```python
from build123d import *

# Parameters (mm, degrees)
F1_DEPTH = 25
F2_W     = 5
F2_H     = 25
F3_DEPTH = 5
F4_SIZE  = 2
F5_R     = 2
F6_R     = 5


with BuildPart() as f1:
    # F0 (on Top) → F1 (new body)
    with BuildSketch(Plane.XY):
        with BuildLine():
            ThreePointArc((57.667806, -47.952312), (0, -75), (-57.667806, -47.952312))
            Line((-57.667806, -47.952312), (-88.564008, -82.249977))
            Line((-88.564008, -82.249977), (0, -82.249977))
            Line((0, -82.249977), (88.564008, -82.249977))
            Line((88.564008, -82.249977), (57.667806, -47.952312))
        make_face()
    extrude(amount=F1_DEPTH)

    # F2 (on face) → F3 (join)
    with BuildSketch(Plane.XZ.offset(82.249977)):
        with Locations((77.608379, 12.5)):
            Rectangle(F2_W, F2_H)
        with Locations((-77.608379, 12.5)):
            Rectangle(F2_W, F2_H)
    extrude(amount=F3_DEPTH)

    # F4
    f4_edges = [f1.edges().sort_by_distance(p)[0] for p in [
        (-80.108379, -87.249977, 12.5),
        (-75.108379, -87.249977, 12.5),
        (75.108379, -87.249977, 12.5),
        (80.108379, -87.249977, 12.5),
    ]]
    chamfer(f4_edges, length=F4_SIZE)

    # F5
    f5_edges = [f1.edges().sort_by_distance(p)[0] for p in [
        (-80.108379, -82.249977, 12.5),
        (-75.108379, -82.249977, 12.5),
        (80.108379, -82.249977, 12.5),
        (75.108379, -82.249977, 12.5),
        (57.667806, -47.952312, 12.5),
        (-57.667806, -47.952312, 12.5),
    ]]
    fillet(f5_edges, radius=F5_R)

    # F6
    f6_edges = [f1.edges().sort_by_distance(p)[0] for p in [
        (-88.564008, -82.249977, 12.5),
        (88.564008, -82.249977, 12.5),
    ]]
    fillet(f6_edges, radius=F6_R)


solid = f1.part
```
Verification items for the finished model (mm, model axes). A direction names the side the tool comes from. Round coordinates to 2 decimals unless told otherwise and drop trailing zeros. Write each loop counter-clockwise with the first axis right and the second up, starting at its lowest first coordinate (ties: lowest second). Pieces come first, ordered by that corner, then holes. Notation, with made-up numbers: (-36.5, -25) -> (8.5, -25) arc R19 cw to (8.5, -4) -> close; hole circle Ø6 at (49.25, 69). An arc over 180 degrees is marked (long way). Write each question's results on one line, items separated by ' | '.
Q1. Sectioned sample at D-D, the plane x = 16.5. Record the boundary of the cut face in (y, z).
Derived:
outline: (-82.25, 0) -> (-73.16, 0) -> (-73.16, 25) -> (-82.25, 25) -> close
Q2. Sectioned sample at B-B, the plane y = -66. Record the boundary of the cut face in (x, z), and give its area (3 significant figures).
Derived:
outline: (-73.93, 0) -> (-35.62, 0) -> (-35.62, 25) -> (-73.93, 25) -> close; (35.62, 0) -> (73.93, 0) -> (73.93, 25) -> (35.62, 25) -> close | area: 1,920 mm²
Q3. Thickness scan on probe 1 along X at (y, z) = (-85, 18.5); probe 2 along X at (y, z) = (-59, 11.75); probe 3 along Y at (x, z) = (-58, 12). Record the ranges inside material, lowest first.
Derived:
probe 1: x = -80.11 to -75.11, 75.11 to 80.11 | probe 2: x = -67.62 to -46.3, 46.3 to 67.62 | probe 3: y = -82.25 to -49
Q4. Draft check along X on faces 1 (the face through (-1, -76, 0)), 2 (the face through (57.672, -48.982, 12.675)), 3 (the face through (70.777, -62.505, 12.325)), 4 (the face through (-70.46, -62.15, 12.32)). Enter one of: released by +X, released by -X, zero draft, split by the parting line, or undercut.
Derived:
face 1: zero draft | face 2: undercut | face 3: released by +X | face 4: released by -X
Q5. Access from +Z, -Z, +X, -X, +Y, -Y to the whole of each face (thin tool, end or side, straight path). Record for faces 5 (the face through (-1, -82.25, 12)), 6 (the face through (0.89, -74.995, 12.325)).
Derived:
face 5: +Z, -Z, -Y | face 6: +Z, -Z, +Y
Q6. Sectioned sample at A-A, the plane y = -53.5. Record the boundary of the cut face in (x, z), and give its area (3 significant figures).
Derived:
outline: (-62.67, 0) -> (-52.56, 0) -> (-52.56, 25) -> (-62.67, 25) -> close; (52.56, 0) -> (62.67, 0) -> (62.67, 25) -> (52.56, 25) -> close | area: 505 mm²
Q7. Go/stop test with flat-tipped pins: pin 1 Ø10 at (y, z) = (-71.5, 13) entering from +X; pin 2 Ø0.8 at (y, z) = (-85, 12.5) entering from -X; pin 3 Ø1.5 at (x, z) = (-65, 14.5) entering from -Y. Record where each tip stops, or that it passes through.
Derived:
pin 1: stops at x = 82.97 | pin 2: stops at x = -80.11 | pin 3: stops at y = -82.25
Q8. Sectioned sample at C-C, the plane x = -36. Record the boundary of the cut face in (y, z).
Derived:
outline: (-82.25, 0) -> (-65.8, 0) -> (-65.8, 25) -> (-82.25, 25) -> close
